Geometry check sheet. Reference: the model listing, model coordinates, mm. Give positions to 0.01 mm unless a question says otherwise; leave off trailing zeros. Loops run counter-clockwise (first coordinate to the right, second up) from the corner with the lowest first, then second, coordinate; pieces in that order, holes last.
```python
from build123d import *

# Parameters (mm, degrees)
F0_W     = 5.225
F0_H     = 5.225
F0_W_2   = 34
F0_H_2   = 34
F1_DEPTH = 3.175
F2_D     = 4.4958
F2_DEPTH = 45.72
F2_TIP   = 1.3506745855
F4_DEPTH = 2
F5_R     = 10.5
F6_DEPTH = 1.176


with BuildPart() as f1:
    # F0 (on Top) → F1 (new body)
    with BuildSketch(Plane.XY):
        Polygon((0, 39.225), (0, 0), (39.225, 0), (39.225, 5.225), (5.225, 5.225), (5.225, 39.225), align=None)
        with Locations((41.8375, 2.6125)):
            Rectangle(F0_W, F0_H)
        with Locations((2.6125, 41.8375)):
            Rectangle(F0_W, F0_H)
        Polygon((39.225, 39.225), (39.225, 5.225), (44.45, 5.225), (44.45, 44.45), (5.225, 44.45), (5.225, 39.225), align=None)
        with Locations((22.225, 22.225)):
            Rectangle(F0_W_2, F0_H_2)
    extrude(amount=F1_DEPTH)

    # F2
    with Locations(Plane(origin=(0, 0, 0), x_dir=(1, 0, 0), z_dir=(0, 0, -1))):
        with Locations((5.225, -39.225), (39.225, -39.225), (39.225, -5.225), (5.225, -5.225)):
            Hole(F2_D / 2, depth=F2_DEPTH)
            with Locations((0, 0, -(F2_DEPTH + F2_TIP / 2))):  # 118° drill point
                Cone(0, F2_D / 2, F2_TIP, mode=Mode.SUBTRACT)

    # F3 (on face) → F4 (cut)
    with BuildSketch(Plane.XY.offset(3.175)):
        with BuildLine():
            ThreePointArc((34.925, 22.225), (31.2052561211, 31.2052561211), (22.225, 34.925))
            Line((22.225, 34.925), (22.225, 22.225))
            Line((22.225, 22.225), (34.925, 22.225))
        make_face()
        with BuildLine():
            Line((22.225, 22.225), (22.225, 34.925))
            ThreePointArc((22.225, 34.925), (13.2447438789, 31.2052561211), (9.525, 22.225))
            Line((9.525, 22.225), (22.225, 22.225))
        make_face()
        with BuildLine():
            Line((34.925, 22.225), (22.225, 22.225))
            Line((22.225, 22.225), (22.225, 9.525))
            ThreePointArc((22.225, 9.525), (31.2052561211, 13.2447438789), (34.925, 22.225))
        make_face()
        with BuildLine():
            Line((22.225, 9.525), (22.225, 22.225))
            Line((22.225, 22.225), (9.525, 22.225))
            ThreePointArc((9.525, 22.225), (13.2447438789, 13.2447438789), (22.225, 9.525))
        make_face()
    extrude(amount=-F4_DEPTH, mode=Mode.SUBTRACT)

    # F5 (on face) → F6 (cut, through all)
    with BuildSketch(Plane.XY.offset(1.175)):
        with Locations((22.225, 22.225)):
            Circle(F5_R)
    extrude(amount=-F6_DEPTH, mode=Mode.SUBTRACT)


solid = f1.part
```
1) Sectioned sample at D-D on y = 19. Enter the section's corners in (x, z) (3 decimals), plus the area to 3 significant figures.
2) Depth check by flat-ended pin: P1, Ø7.5, axis at x = 24.5, y = 17.5, coming from the +Z side (3 decimals); P2, Ø10, axis at x = 15.5, y = 22, coming from the +Z side (3 decimals). Enter the tip coordinate at first touch or a pass-through.
3) Sectioned sample at B-B on x = 20.5. Enter the section's corners in (y, z) (3 decimals), plus the area to 3 significant figures.
4) Mould release check, pull along Y, two halves, no side actions. Record for faces 1 (the flat face through (23, 44.45, 2)), 2 (the flat face through (32, 27, 0)), 3 (the flat face through (17, 32, 1.175)): +Y half, -Y half, draft (parallel to the pull), parting line (faces both ways), or undercut.
5) Sectioned sample at C-C on z = 2. Enter the section's corners in (x, y) (3 decimals), plus the area to 3 significant figures.
6) Sectioned sample at A-A on y = 6.5. Enter the section's corners in (x, z) (3 decimals), plus the area to 3 significant figures.
7) Scan lines: line 1 along X through (y, z) = (39, 2.9); line 2 along Y through (x, z) = (3.5, 1.4); line 3 along Z through (x, y) = (17, 12.5) (3 decimals). Record each from-to range of solid material in increasing order.
Determined:
1. outline: (0, 0) - (12.233, 0) - (12.233, 1.175) - (9.941, 1.175) - (9.941, 3.175) - (0, 3.175) - close; (32.217, 0) - (44.45, 0) - (44.45, 3.175) - (34.509, 3.175) - (34.509, 1.175) - (32.217, 1.175) - close
1. area: 68.5 mm2
2. P1: passes through
2. P2: stops at z = 1.175
3. outline: (0, 0) - (11.868, 0) - (11.868, 1.175) - (9.643, 1.175) - (9.643, 3.175) - (0, 3.175) - close; (32.582, 0) - (44.45, 0) - (44.45, 3.175) - (34.807, 3.175) - (34.807, 1.175) - (32.582, 1.175) - close
3. area: 66.5 mm2
4. face 1: +Y half
4. face 2: draft
4. face 3: undercut
5. outline: (0, 0) - (44.45, 0) - (44.45, 44.45) - (0, 44.45) - close; hole circle Ø4.496 at (5.225, 5.225); hole circle Ø4.496 at (5.225, 39.225); hole circle Ø25.4 at (22.225, 22.225); hole circle Ø4.496 at (39.225, 5.225); hole circle Ø4.496 at (39.225, 39.225)
5. area: 1,410 mm2
6. outline: (0, 0) - (3.374, 0) - (3.374, 3.175) - (0, 3.175) - close; (7.076, 0) - (37.374, 0) - (37.374, 3.175) - (7.076, 3.175) - close; (41.076, 0) - (44.45, 0) - (44.45, 3.175) - (41.076, 3.175) - close
6. area: 118 mm2
7. line 1: x = 0 to 2.99, 7.46 to 36.99, 41.46 to 44.45
7. line 2: y = 0 to 3.78, 6.67 to 37.78, 40.67 to 44.45
7. line 3: z = 0 to 1.175
